Input: part model. Units: mm. Frame: model coordinates. Face numbers are marked on the shaded views. A direction names the side the tool comes from. Give positions to 0.01 mm unless a question says otherwise; leave off trailing zeros. Order: outer loops, then holes, each group sorted by start corner. A loop starts at its lowest first (then second) coordinate and runs counter-clockwise, first axis right, second up. Notation, with made-up numbers: (-36.5, 13.25) - (-20.5, 13.25) arc R25 ccw to (-20.5, 33.25) - close; hole circle Ø2 at (5.5, 73). An arc over 180 degrees is marked (long way). Answer in a Markdown table with one row per item. Add a question column.
from build123d import *

# Parameters (mm, degrees)
SKETCH1_W                                      = 50
SKETCH1_H                                      = 50
BOSS_EXTRUDE1_DEPTH                            = 40
SHELL1_T                                       = -2.5
BOSS_EXTRUDE5_DEPTH                            = 18
SKETCH17_W                                     = 22.5
SKETCH17_H                                     = 6.5
BOSS_EXTRUDE6_DEPTH                            = 8
SKETCH18_W                                     = 6.5
SKETCH18_H                                     = 29.5
BOSS_EXTRUDE7_DEPTH                            = 8
SKETCH19_W                                     = 11
SKETCH19_H                                     = 30.2
CUT_EXTRUDE5_DEPTH                             = 6.2
SKETCH20_W                                     = 30.2
SKETCH20_H                                     = 5.4
CUT_EXTRUDE6_DEPTH                             = 6.2
SKETCH21_W                                     = 5
SKETCH21_H                                     = 5
BOSS_EXTRUDE8_DEPTH                            = 8
CSK_SLOT_FOR_M1_6_COUNTERSUNK_FLAT_H_2_COUNT   = 2
CSK_SLOT_FOR_M1_6_COUNTERSUNK_FLAT_H_2_PITCH   = 22
SKETCH28_R                                     = 3
CUT_EXTRUDE7_DEPTH                             = 47.046172479
CSK_SLOT_FOR_M1_6_COUNTERSUNK_FLAT_H_3_A_COUNT = 2
CSK_SLOT_FOR_M1_6_COUNTERSUNK_FLAT_H_3_A_PITCH = 22
SKETCH32_R                                     = 3
CUT_EXTRUDE8_DEPTH                             = 62.524385409
CUT_EXTRUDE10_REACH                            = 48.046
SKETCH34_W                                     = 6
SKETCH34_H                                     = 6.5
SKETCH35_W                                     = 5
SKETCH35_H                                     = 5
BOSS_EXTRUDE9_DEPTH                            = 8
CSK_SLOT_FOR_M2_COUNTERSUNK_FLAT_HEA_2_COUNT   = 2
CSK_SLOT_FOR_M2_COUNTERSUNK_FLAT_HEA_2_PITCH   = 29.99
CSK_SLOT_FOR_M2_COUNTERSUNK_FLAT_HEA_3_COUNT   = 2
CSK_SLOT_FOR_M2_COUNTERSUNK_FLAT_HEA_3_PITCH   = 16
CSK_SLOT_FOR_M2_COUNTERSUNK_FLAT_HEA_4_COUNT   = 2
CSK_SLOT_FOR_M2_COUNTERSUNK_FLAT_HEA_4_PITCH   = 33.991176796
SKETCH38_W                                     = 13
SKETCH38_H                                     = 10
CUT_EXTRUDE11_DEPTH                            = 10


with BuildPart() as part:
    # Sketch1 → Boss-Extrude1 (new body)
    with BuildSketch(Plane(origin=(0, 0, 0), x_dir=(1, 0, 0), z_dir=(0, 1, 0))):
        Rectangle(SKETCH1_W, SKETCH1_H)
    extrude(amount=BOSS_EXTRUDE1_DEPTH)

    # Shell1
    shell1_openings = [part.faces().sort_by_distance(p)[0] for p in [
        (0, 40, 0),
    ]]
    offset(amount=SHELL1_T, openings=shell1_openings, kind=Kind.INTERSECTION)

    # Sketch16 → Boss-Extrude5 (add)
    with BuildSketch(Plane(origin=(0, 2.5, 0), x_dir=(1, 0, 0), z_dir=(0, 1, 0))):
        Polygon((-10.3, 6.5), (-22.5, 6.5), (-22.5, 22.5), (-5.169122612, 22.5), (22.5, 22.5), (22.5, 6.5), (10.3, 6.5), (10.3, 13.5), (-5.169122612, 13.5), (-10.3, 13.5), align=None)
        Polygon((10.3, -13.6), (22.5, -13.6), (22.5, -22.5), (-4.979068663, -22.5), (-22.5, -22.5), (-22.5, -13.6), (-10.3, -13.6), (-10.3, -20.79), (-4.979068663, -20.79), (10.3, -20.79), align=None)
    extrude(amount=BOSS_EXTRUDE5_DEPTH)

    # Sketch17 → Boss-Extrude6 (add)
    with BuildSketch(Plane(origin=(0, 2.5, 0), x_dir=(1, 0, 0), z_dir=(0, 1, 0))):
        Polygon((0, 0), (0, 6.5), (-10.3, 6.5), (-22.5, 6.5), (-22.5, 0), align=None)
        with Locations((-11.25, -3.25)):
            Rectangle(SKETCH17_W, SKETCH17_H)
        Polygon((10.3, 6.5), (0, 6.5), (0, 0), (0, -6.5), (22.5, -6.5), (22.5, 6.5), align=None)
    extrude(amount=BOSS_EXTRUDE6_DEPTH)

    # Sketch18 → Boss-Extrude7 (add)
    with BuildSketch(Plane(origin=(-22.5, 0, 0), x_dir=(0, 0, -1), z_dir=(1, 0, 0))):
        Polygon((6.5, 40), (0, 40), (0, 10.5), (6.5, 10.5), (6.5, 20.5), align=None)
        with Locations((-3.25, 25.25)):
            Rectangle(SKETCH18_W, SKETCH18_H)
    extrude(amount=BOSS_EXTRUDE7_DEPTH)

    # Sketch19 → Cut-Extrude5 (cut)
    with BuildSketch(Plane.ZY.offset(25)):
        with Locations((0, 24.9)):
            Rectangle(SKETCH19_W, SKETCH19_H)
    extrude(amount=-CUT_EXTRUDE5_DEPTH, mode=Mode.SUBTRACT)

    # Sketch20 → Cut-Extrude6 (cut)
    with BuildSketch(Plane.XZ):
        with Locations((0, 2.7)):
            Rectangle(SKETCH20_W, SKETCH20_H)
        with Locations((0, -2.7)):
            Rectangle(SKETCH20_W, SKETCH20_H)
    extrude(amount=-CUT_EXTRUDE6_DEPTH, mode=Mode.SUBTRACT)

    # Sketch21 → Boss-Extrude8 (add)
    with BuildSketch(Plane(origin=(0, 2.5, 0), x_dir=(1, 0, 0), z_dir=(0, 1, 0))):
        with Locations((7.8, -18.29)):
            Rectangle(SKETCH21_W, SKETCH21_H)
        with Locations((-7.8, -18.29)):
            Rectangle(SKETCH21_W, SKETCH21_H)
    extrude(amount=BOSS_EXTRUDE8_DEPTH)

    # Sketch26 → CSK SLOT for M1.6 Countersunk Flat Head (revolve, cut)
    with BuildSketch(Plane(origin=(-11, 10.5, 0), x_dir=(0, 0, 1), z_dir=(1, 0, 0))):
        Polygon((0, 0), (0, 10.5), (0.9, 10.5), (0.9, 3.9), (1.8, 3), (1.8, 0), align=None)
    csk_slot_for_m1_6_countersunk_flat_head = revolve(axis=Axis((-11, 16.85, 0), (0, -1, 0)), mode=Mode.SUBTRACT)

    # CSK SLOT for M1.6 Countersunk Flat H 2: CSK SLOT for M1.6 Countersunk Flat Head ×2
    with Locations(*[(i * CSK_SLOT_FOR_M1_6_COUNTERSUNK_FLAT_H_2_PITCH, 0, 0) for i in range(1, CSK_SLOT_FOR_M1_6_COUNTERSUNK_FLAT_H_2_COUNT)]):
        add(csk_slot_for_m1_6_countersunk_flat_head, mode=Mode.SUBTRACT)

    # Sketch28 → Cut-Extrude7 (cut, through all)
    with BuildSketch(Plane(origin=(0, 10.5, 0), x_dir=(1, 0, 0), z_dir=(0, 1, 0))):
        with Locations(Location((0, 0, 0), (0, 0, 270))):
            Circle(SKETCH28_R)
    extrude(amount=-CUT_EXTRUDE7_DEPTH, mode=Mode.SUBTRACT)

    # Sketch31 → CSK SLOT for M1.6 Countersunk Flat H 3 (revolve, cut)
    with BuildSketch(Plane(origin=(-14.5, 36, 0), x_dir=(0, 0, -1), z_dir=(0, 1, 0))):
        Polygon((0, 0), (0, 10.5), (0.9, 10.5), (0.9, 3.9), (1.8, 3), (1.8, 0), align=None)
    csk_slot_for_m1_6_countersunk_flat_h_3 = revolve(axis=Axis((-8.15, 36, 0), (-1, 0, 0)), mode=Mode.SUBTRACT)

    # CSK SLOT for M1.6 Countersunk Flat H 3 a: CSK SLOT for M1.6 Countersunk Flat H 3 ×2
    with Locations(*[(0, -i * CSK_SLOT_FOR_M1_6_COUNTERSUNK_FLAT_H_3_A_PITCH, 0) for i in range(1, CSK_SLOT_FOR_M1_6_COUNTERSUNK_FLAT_H_3_A_COUNT)]):
        add(csk_slot_for_m1_6_countersunk_flat_h_3, mode=Mode.SUBTRACT)

    # Sketch32 → Cut-Extrude8 (cut, through all)
    with BuildSketch(Plane(origin=(-14.5, 0, 0), x_dir=(0, 0, -1), z_dir=(1, 0, 0))):
        with Locations((0, 25)):
            Circle(SKETCH32_R)
    extrude(amount=-CUT_EXTRUDE8_DEPTH, mode=Mode.SUBTRACT)

    # Cut-Extrude10: up to this face of the body (flat: up to its plane)
    cut_extrude10_end = Plane(part.part.faces().sort_by_distance((0, 2.5, 11.597540384))[0])
    # Sketch34 → Cut-Extrude10 (cut, up to the picked face)
    with BuildSketch(Plane(origin=(0, 10.5, 0), x_dir=(1, 0, 0), z_dir=(0, 1, 0)), mode=Mode.PRIVATE) as cut_extrude10_sk1:
        with Locations((0, -3.25)):
            Rectangle(SKETCH34_W, SKETCH34_H)
    cut_extrude10_tool1 = split(extrude(cut_extrude10_sk1.sketch, amount=-CUT_EXTRUDE10_REACH, mode=Mode.PRIVATE), bisect_by=cut_extrude10_end, keep=Keep.BOTH, mode=Mode.PRIVATE)
    add(cut_extrude10_tool1.solids().sort_by(Axis((0, 10.5, 3.25), (0, -1, 0)))[0], mode=Mode.SUBTRACT)

    # Sketch35 → Boss-Extrude9 (add)
    with BuildSketch(Plane(origin=(0, 2.5, 0), x_dir=(1, 0, 0), z_dir=(0, 1, 0))):
        with Locations((-7.8, 11)):
            Rectangle(SKETCH35_W, SKETCH35_H)
        with Locations((7.8, 11)):
            Rectangle(SKETCH35_W, SKETCH35_H)
    extrude(amount=BOSS_EXTRUDE9_DEPTH)

    # Sketch37 → CSK SLOT for M2 Countersunk Flat Head Screw1 (revolve, cut)
    with BuildSketch(Plane(origin=(8, 0, 18.64), x_dir=(0, 0, -1), z_dir=(1, 0, 0))):
        Polygon((0, 0), (0, 40), (1.2, 40), (1.2, 10), (2.2, 9), (2.2, 0), align=None)
    csk_slot_for_m2_countersunk_flat_head_sc = revolve(axis=Axis((8, -6.35, 18.64), (0, 1, 0)), mode=Mode.SUBTRACT)

    # CSK SLOT for M2 Countersunk Flat Hea 2: CSK SLOT for M2 Countersunk Flat Head Screw1 ×2
    with Locations(*[(0, 0, -i * CSK_SLOT_FOR_M2_COUNTERSUNK_FLAT_HEA_2_PITCH) for i in range(1, CSK_SLOT_FOR_M2_COUNTERSUNK_FLAT_HEA_2_COUNT)]):
        add(csk_slot_for_m2_countersunk_flat_head_sc, mode=Mode.SUBTRACT)

    # CSK SLOT for M2 Countersunk Flat Hea 3: CSK SLOT for M2 Countersunk Flat Head Screw1 ×2
    with Locations(*[(-i * CSK_SLOT_FOR_M2_COUNTERSUNK_FLAT_HEA_3_PITCH, 0, 0) for i in range(1, CSK_SLOT_FOR_M2_COUNTERSUNK_FLAT_HEA_3_COUNT)]):
        add(csk_slot_for_m2_countersunk_flat_head_sc, mode=Mode.SUBTRACT)

    # CSK SLOT for M2 Countersunk Flat Hea 4: CSK SLOT for M2 Countersunk Flat Head Screw1 ×2
    with Locations(*[Vector(-0.47071038745922766, 0, -0.882287782493889) * (i * CSK_SLOT_FOR_M2_COUNTERSUNK_FLAT_HEA_4_PITCH) for i in range(1, CSK_SLOT_FOR_M2_COUNTERSUNK_FLAT_HEA_4_COUNT)]):
        add(csk_slot_for_m2_countersunk_flat_head_sc, mode=Mode.SUBTRACT)

    # Sketch38 → Cut-Extrude11 (cut)
    with BuildSketch(Plane.ZY.offset(-22.5)):
        with Locations((0, 15.5)):
            Rectangle(SKETCH38_W, SKETCH38_H)
    extrude(amount=-CUT_EXTRUDE11_DEPTH, mode=Mode.SUBTRACT)


solid = part.part
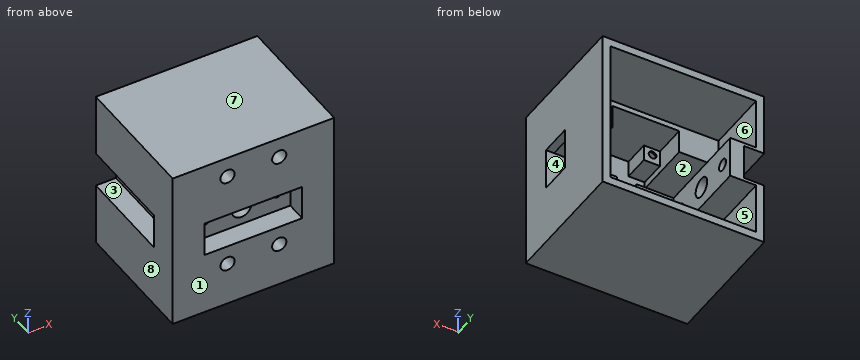
Q1. Section B-B, the plane z = -11.35. State how many separate pieces and enclosed holes the cut face has, then the cut area to 3 significant figures.
Q2. Access query for the marked faces 1, 2, 3 and 4. Directions: +Z, -Z, +X, -X, +Y, -Y. A direction counts if a zero-diameter tool reaches every point of the face in a straight line with its end or side. Return the directions, or none.
Q3. Section C-C, the plane y = 32. Return loops of the section in (x, z).
Q4. Line query: probe 1 along Z at (x, y) = (8, 10.25); probe 2 along X at (y, z) = (3, -11.35); probe 3 along Z at (x, y) = (11, 4.5). Output: solid intervals per line, ascending.
Q5. Section A-A, the plane x = 11. Return loops of the section in (y, z).
Q6. Contact query for flat-ended pins moving along their axis: P1, Ø1.5, axis at x = 7, z = 18, coming from the +Y side; P2, Ø3, axis at y = 14, z = 0, coming from the +X side; P3, Ø2, axis at x = 8, z = -11.35, coming from the -Y side. Output: stop coordinate, or through.
Q7. Section D-D, the plane z = 21.5. Return loops of the section in (x, y), then the cut area to 3 significant figures.
Q8. Pull-direction query (X, two-part tool) for the marked faces 5, 6, 7 and 8; classes: +X half, -X half, draft (parallel to the pull), parting line (faces both ways), or undercut.
Computed:
| question | item | result |
|---|---|---|
| 1 | separate pieces | 3 |
| 1 | enclosed holes | 0 |
| 1 | area | 743 mm^2 |
| 2 | face 1 | +Z, -Z, +X, -X, -Y |
| 2 | face 2 | +Y |
| 2 | face 3 | -X, +Y |
| 2 | face 4 | +X |
| 3 | outline | (-25, -25) - (25, -25) - (25, 25) - (-25, 25) - (-25, 5.5) - (-18.8, 5.5) - (-18.8, -5.5) - (-25, -5.5) - close; hole (-22.5, -22.5) - (22.5, -22.5) - (22.5, 22.5) - (-22.5, 22.5) - (-22.5, 6.5) - (-14.5, 6.5) - (-14.5, -6.5) - (-22.5, -6.5) - close |
| 4 | probe 1 | z = -25 to -12.55, -10.15 to -8.5, -6.5 to 6.5, 15.79 to 17.44, 19.84 to 25 |
| 4 | probe 2 | x = -25 to -10.2, -5.8 to -5.3, 5.3 to 5.8, 10.2 to 25 |
| 4 | probe 3 | z = -25 to -5.4, 5.4 to 6.5, 13.6 to 25 |
| 5 | outline | (0, -25) - (40, -25) - (40, -22.5) - (20.5, -22.5) - (20.5, -6.5) - (10.5, -6.5) - (10.5, -1.8) - (7.5, -1.8) - (6.6, -0.9) - (6.2, -0.9) - (6.2, -5.4) - (0, -5.4) - close; (0, 5.4) - (6.2, 5.4) - (6.2, 0.9) - (6.6, 0.9) - (7.5, 1.8) - (10.5, 1.8) - (10.5, 6.5) - (2.5, 6.5) - (2.5, 13.6) - (20.5, 13.6) - (20.5, 22.5) - (40, 22.5) - (40, 25) - (0, 25) - close |
| 6 | P1 | stops at y = 10.5 |
| 6 | P2 | stops at x = -17.8 |
| 6 | P3 | passes through |
| 7 | outline | (-25, 0) - (25, 0) - (25, 40) - (22.5, 40) - (22.5, 20.5) - (-22.5, 20.5) - (-22.5, 40) - (-25, 40) - close |
| 7 | area | 1,120 mm^2 |
| 8 | face 5 | undercut |
| 8 | face 6 | undercut |
| 8 | face 7 | draft |
| 8 | face 8 | -X half |
